Input: part model. Units: mm. Frame: model coordinates. Face numbers are marked on the shaded views. A direction names the side the tool comes from. Coordinates: 2 decimals unless noted, no trailing zeros. Write each loop counter-clockwise with the first axis right and the second up, starting at its lowest first coordinate (ties: lowest second). Pieces come first, ordered by that corner, then holes. Notation, with made-up numbers: M 74,66.25 L 109,66.25 A11 cw 109,76.25 Z; hole C 2.5,68 d1. An arc over 180 degrees is marked long. Use one line per item in the form item = value.
from build123d import *

# Parameters (mm, degrees)
SKETCH_1_R      = 3.5
EXTRUDE_1_DEPTH = 2.5
SKETCH_2_R      = 2
EXTRUDE_2_DEPTH = 20
EXTRUDE_3_DEPTH = 1


with BuildPart() as part:
    # 草图1 → 凸台-拉伸1 (new body)
    with BuildSketch(Plane.XY):
        Circle(SKETCH_1_R)
        Polygon((2.020725942, 0), (1.010362971, 1.75), (-1.010362971, 1.75), (-2.020725942, 0), (-1.010362971, -1.75), (1.010362971, -1.75), align=None, mode=Mode.SUBTRACT)
    extrude(amount=EXTRUDE_1_DEPTH)

    # 草图2 → 凸台-拉伸2 (add)
    with BuildSketch(Plane(origin=(0, 0, 0), x_dir=(-1, 0, 0), z_dir=(0, 0, -1))):
        with Locations(Location((0, 0, 0), (0, 0, 178.955024372))):
            Circle(SKETCH_2_R)
    extrude(amount=EXTRUDE_2_DEPTH)

    # 草图1<3> → 凸台-拉伸3 (add)
    with BuildSketch(Plane.XY):
        Polygon((-1.010362971, -1.75), (1.010362971, -1.75), (2.020725942, 0), (1.010362971, 1.75), (-1.010362971, 1.75), (-2.020725942, 0), align=None)
    extrude(amount=EXTRUDE_3_DEPTH)


solid = part.part
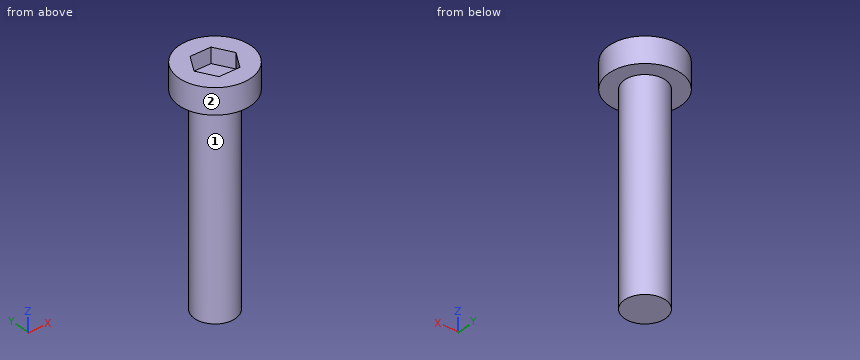
(1) Section query B-B on y = -1. Return the cut outline in (x, z).
Computed:
outline = M -3.35,0 L -1.73,0 L -1.73,-20 L 1.73,-20 L 1.73,0 L 3.35,0 L 3.35,2.5 L 1.44,2.5 L 1.44,1 L -1.44,1 L -1.44,2.5 L -3.35,2.5 Z
(2) First-contact query: pin 1 Ø1.5 at (x, y) = (-2, -2) entering from -Z; pin 2 Ø2 at (y, z) = (0.5, -14) entering from +X. Flat tips, straight axial feed; report the tip coordinate or a pass-through.
Computed:
pin_1 = 0
pin_2 = 2
(3) Set-up query: the marked faces 1 and 2. Return all of +Z, -Z, +X, -X, +Y, -Y with unobstructed straight access to the full face (end or side cutting, diameter ignored); none if empty.
Computed:
face_1 = -Z
face_2 = +Z, -Z
(4) Section query C-C on z = 0.5. Return the cut outline in (x, y).
Computed:
outline = C 0,0 d7
(5) Section query A-A on x = 0. Return the cut outline in (y, z), plus the area to 4 significant figures.
Computed:
outline = M -3.5,0 L -2,0 L -2,-20 L 2,-20 L 2,0 L 3.5,0 L 3.5,2.5 L 1.75,2.5 L 1.75,1 L -1.75,1 L -1.75,2.5 L -3.5,2.5 Z
area = 92.25 mm^2
(6) Section query D-D on z = -13.75. Return the cut outline in (x, y), plus the area to 3 significant figures.
Computed:
outline = C 0,0 d4
area = 12.6 mm^2
(7) Line query: probe 1 along Z at (x, y) = (2, -1.5); probe 2 along Y at (x, z) = (0, -4). Output: solid intervals per line, ascending.
Computed:
probe_1 = 0 to 2.5
probe_2 = -2 to 2
